Input: part model. Units: mm. Frame: model coordinates. Face numbers are marked on the shaded views. A direction names the side the tool comes from. Round coordinates to 2 decimals unless told otherwise and drop trailing zeros. Loops run counter-clockwise (first coordinate to the right, second up) from the corner with the lowest first, then second, coordinate; pieces in that order, holes last.
1) Section B-B, the plane x = 147.5. Return loops of the section in (y, z), and give its area (3 significant figures).
2) Section A-A, the plane z = -6.75. Return loops of the section in (x, y) (3 decimals).
3) Access query for the marked faces 4 and 5. Directions: +Z, -Z, +X, -X, +Y, -Y. A direction counts if a zero-diameter tool reaches every point of the face in a straight line with its end or side. Return the directions, or none.
4) Draft query along X for the marked faces 1, 2 and 3. Return one class per face: pulls with the +X half, pulls with the -X half, needs draft (parallel to the pull), parting line crosses it, or undercut.
5) First-contact query: pin 1 (3 mm diameter, centred on y = 3, z = -13.5, fed in from +X); pin 2 (4 mm diameter, centred on y = 11, z = -2.5, fed in from +X). Flat tips, straight axial feed; report the tip coordinate or a pass-through.
6) Ray query, line 1 along Y through (x, z) = (57, 0); line 2 along X through (y, z) = (17, -14.5); line 3 along X through (y, z) = (18, -2.25). Return the intervals inside material, ascending.
Autodesk Inventor part; units mm, degrees
ref_plane "YZ Plane" through (0, 0, 0) normal (1, 0, 0) x (0, 1, 0)
ref_plane "XZ Plane" through (0, 0, 0) normal (0, 1, 0) x (-1, 0, 0)
ref_plane "XY Plane" through (0, 0, 0) normal (0, 0, 1) x (1, 0, 0)
sketch "Sketch1" plane through (0, 0, 0) normal (0, 0, 1) x (1, 0, 0)
  line L0 (0, 0) -> (170.6562, 0)
  line L1 (170.6562, 33.7312) -> (0, 33.7312)
  arc A0 (0, 33.7312) -> (0, 0) centre (0, 16.8656) ccw
  arc A1 (170.6562, 0) -> (170.6562, 33.7312) centre (170.6562, 16.8656) ccw
  dimension "d2" = 16.8656
  dimension "d3" = 170.6562
sketch "Sketch2" plane through (0, 0, 0) normal (1, 0, 0) x (0, 1, 0)
  arc A0 (0.9906, 0) -> (-0.9906, 0) centre (0, 0) ccw
  line L0 (-0.9906, 0) -> (0.9906, 0) construction
  line L1 (-0.9906, 0) -> (-0.9906, -17.0688)
  line L2 (0.9906, 0) -> (0.9906, -17.0688)
  arc A1 (-0.9906, -17.0688) -> (0.9906, -17.0688) centre (0, -17.0688) ccw
  dimension "d8" = 1.9812
  dimension "d9" = 19.05
sweep "Sweep1" add profiles "Sketch2" path "Sketch1"
properties part number "Polycord" material "Rubber, Silicone"
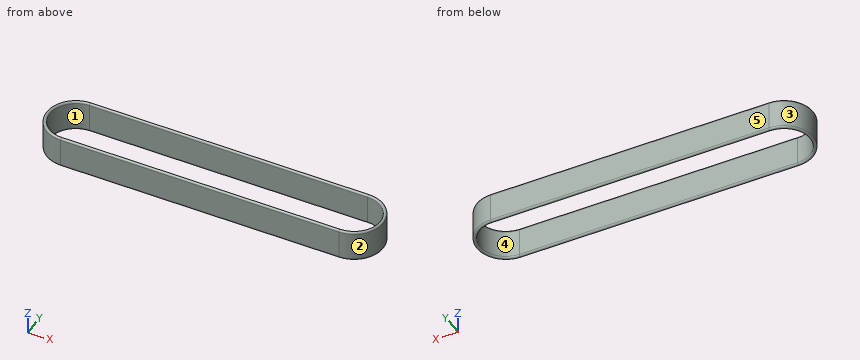
Final values:
1. outline: (-0.99, -17.07) arc R0.99 ccw to (0.99, -17.07) - (0.99, 0) arc R0.99 ccw to (-0.99, 0) - close; (32.74, -17.07) arc R0.99 ccw to (34.72, -17.07) - (34.72, 0) arc R0.99 ccw to (32.74, 0) - close
1. area: 73.8 mm2
2. outline: (0, -0.991) - (170.656, -0.991) arc R17.856 ccw to (170.656, 34.722) - (0, 34.722) arc R17.856 ccw to start; hole (0, 0.991) - (170.656, 0.991) arc R15.875 ccw to (170.656, 32.741) - (0, 32.741) arc R15.875 ccw to start
3. face 4: +Z, -Z
3. face 5: +Z, -Z, +X, -X, +Y
4. face 1: undercut
4. face 2: pulls with the +X half
4. face 3: pulls with the -X half
5. pin 1: stops at x = 183.54
5. pin 2: stops at x = 188.09
6. line 1: y = -0.99 to 0.99, 32.74 to 34.72
6. line 2: x = -17.86 to -15.87, 186.53 to 188.51
6. line 3: x = -17.82 to -15.83, 186.49 to 188.48
